Geometry check sheet. Reference: the model listing, model coordinates, mm. Face numbers are marked on the shaded views. A direction names the side the tool comes from. Round coordinates to 2 decimals unless told otherwise and drop trailing zeros. Write each loop counter-clockwise with the first axis right and the second up, starting at its lowest first coordinate (ties: lowest second). Pieces come first, ordered by that corner, then holes. Notation, with made-up numbers: (62.5, 59) - (80.5, 59) arc R22 ccw to (80.5, 71) - close; hole circle Ø10 at (56, 30.25). An arc over 180 degrees is marked (long way). Return JSON: item names as keys, results as strings.
```python
from build123d import *

# Parameters (mm, degrees)
F0_W     = 9.5021461621
F0_H     = 2.6417713279
F2_DEPTH = 10
F1_R     = 4.25
F4_DEPTH = 10


with BuildPart() as f2:
    # F0 (on Front) → F2 (new body)
    with BuildSketch(Plane.XZ):
        Polygon((-1.2758228406, -32.4617078483), (-1.2758228406, -35.7812091163), (7.6683001402, -35.7812091163), (7.6683001402, -19.8199365203), (-47.2758228406, -19.8199365203), (-47.2758228406, -22.4617078483), (5.7241771594, -22.4617078483), (5.7241771594, -34.4617078483), (0.7241771594, -34.4617078483), (0.7241771594, -32.4617078483), align=None)
        with Locations((-52.0268959217, -21.1408221843)):
            Rectangle(F0_W, F0_H)
        Polygon((-47.2758228406, -32.4617078483), (-47.2758228406, -22.4617078483), (-56.7779690027, -22.4617078483), align=None)
    extrude(amount=F2_DEPTH)



with BuildPart() as f2b:
    # F1 (on Front) → F2, piece 2 (new body)
    with BuildSketch(Plane.XZ):
        with BuildLine():
            Line((-145.7300181234, 65.3582332276), (-56.7768959217, -22.4617078483))
            Line((-56.7768959217, -22.4617078483), (-40.5840538442, -20.1916061342))
            Line((-40.5840538442, -20.1916061342), (-136.6024373877, 74.6035913392))
            ThreePointArc((-136.6024373877, 74.6035913392), (-140.1472862331, 76.0453637221), (-143.6733599188, 74.5582640942))
            Line((-143.6733599188, 74.5582640942), (-145.7753453684, 72.4291557587))
            ThreePointArc((-145.7753453684, 72.4291557587), (-147.2171177514, 68.8843069133), (-145.7300181234, 65.3582332276))
        make_face()
        with Locations((-139.9780238936, 68.6254584758)):
            Circle(F1_R, mode=Mode.SUBTRACT)
    extrude(amount=F2_DEPTH)


with BuildPart() as f2_1:
    add(f2.part)

    add(f2b.part)  # F4 merges F2b
    # F3 (on Front) → F4 (join)
    with BuildSketch(Plane.XZ):
        Polygon((-2.4996690918, -20.4601678997), (-118.4480087704, 53.6740520599), (-116.2248924375, 46.2126098573), (-11.9464918971, -20.4601678997), align=None)
    extrude(amount=F4_DEPTH)


solid = f2_1.part
```
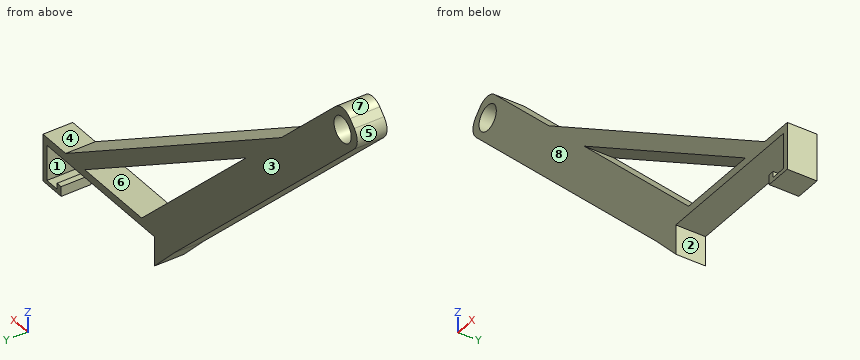
(1) Material ranges on line 1 along X through (y, z) = (-2, -22.5); line 2 along Z through (x, y) = (-1.5, -8.25); line 3 along Z through (x, y) = (-30.5, -5), recorded low to high. Write a range as [from, to].
Response values:
{"line 1": "x = [-56.74, -47.28], [5.72, 7.67]", "line 2": "z = [-22.46, -19.82]", "line 3": "z = [-22.46, -19.82], [-8.6, -2.56]"}
(2) Access from +Z, -Z, +X, -X, +Y, -Y to the whole of each face (thin tool, end or side, straight path). Record for the marked faces 1, 2, 3 and 4.
Response values:
{"face 1": "+Y, -Y", "face 2": "-Z, +Y, -Y", "face 3": "+Z, -Z, +X, -X, +Y", "face 4": "+Z, +X, +Y, -Y"}
(3) Section check A-A, the plane z = 13.5. Enter the section's corners in (x, y).
Response values:
{"outline": "(-93.2, -10) - (-74.71, -10) - (-74.71, 0) - (-93.2, 0) - close; (-65.06, -10) - (-55.61, -10) - (-55.61, 0) - (-65.06, 0) - close"}
(4) Section check D-D, the plane x = -116.5. Enter the section's corners in (y, z), plus the area to 3 significant figures.
Response values:
{"outline": "(-10, 36.5) - (0, 36.5) - (0, 54.76) - (-10, 54.76) - close", "area": "183 mm^2"}
(5) Gauge pin test, flat ends, axial feed: pin 1 (7.5 mm diameter, centred on x = -139.98, z = 68.63, fed in from +Y); pin 2 (3 mm diameter, centred on x = -29.5, y = -3, fed in from -Z); pin 3 (2.5 mm diameter, centred on x = 2, y = -6, fed in from +Z); pin 4 (2 mm diameter, centred on x = -46.5, y = -4, fed in from +Z). Record the tip position at first contact, or that the pin passes through.
Response values:
{"pin 1": "passes through", "pin 2": "stops at z = -22.46", "pin 3": "stops at z = -19.82", "pin 4": "stops at z = 8.31"}
(6) Section check B-B, the plane x = -15. Enter the section's corners in (y, z).
Response values:
{"outline": "(-10, -22.46) - (0, -22.46) - (0, -19.82) - (-10, -19.82) - close; (-10, -18.51) - (0, -18.51) - (0, -12.47) - (-10, -12.47) - close"}
(7) Release check for a two-part mould opening along Z. For the marked faces 5, 6, 7 and 8 record: pulls with the +Z half, pulls with the -Z half, needs draft (parallel to the pull), parting line crosses it, or undercut.
Response values:
{"face 5": "parting line crosses it", "face 6": "undercut", "face 7": "pulls with the +Z half", "face 8": "needs draft"}
(8) Section check C-C, the plane y = -3.5. Give the number of separate pieces and of enclosed holes in the cut face, plus the area to 3 significant figures.
Response values:
{"separate pieces": "1", "enclosed holes": "2", "area": "2,480 mm^2"}
